Autodesk Inventor part; units mm, degrees
ref_plane "YZ Plane" through (0, 0, 0) normal (1, 0, 0) x (0, 1, 0)
ref_plane "XZ Plane" through (0, 0, 0) normal (0, 1, 0) x (-1, 0, 0)
ref_plane "XY Plane" through (0, 0, 0) normal (0, 0, 1) x (1, 0, 0)
sketch "Sketch1" plane through (0, 0, 0) normal (0, 1, 0) x (-1, 0, 0)
  line L0 (10.0011, -4.0004) -> (-4.061, -4.0004)
  line L1 (-4.061, -4.0004) -> (-4.061, -20.083)
  line L2 (-4.061, -20.083) -> (0, -13.9813)
  line L3 (0, -13.9813) -> (0, -8.1221)
  line L4 (0, -8.1221) -> (10.0011, -8.1221)
  line L5 (10.0011, -8.1221) -> (10.0011, -4.0004)
  line L6 (12.8135, 0) -> (-6.8735, 0)
  point P0 (0, 0)
revolve "Revolution1" add sketch "Sketch1" angle 360 about axis through (-10, 0, 0) along (1, 0, 0)
fillet "Fillet1" radius 2 1 edges at (4.061, 0, 20.083)
fillet "Fillet2" radius 2 2 edges at (-10.0011, 0, 8.1221) (0, 0, 8.1221)
properties part number "revolution_example"
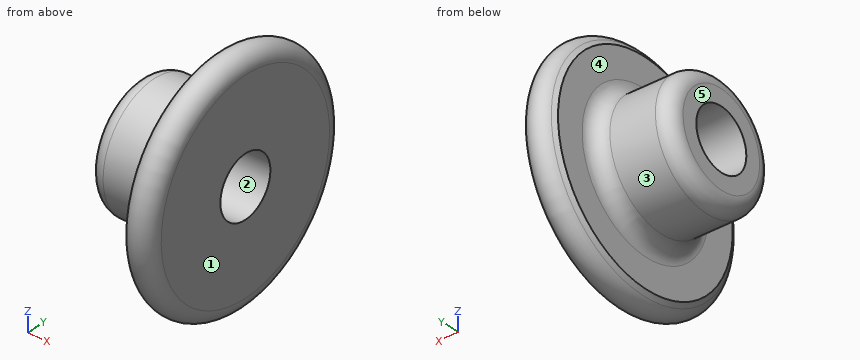
The model under review builds one solid part; all positions refer to its coordinate system, in mm. Face numbers are marked on the shaded views. A direction names the side the tool comes from. Round coordinates to 2 decimals unless told otherwise and drop trailing zeros. Write each loop counter-clockwise with the first axis right and the second up, starting at its lowest first coordinate (ties: lowest second). Pieces come first, ordered by that corner, then holes.
(1) We need section C-C on x = -3.25. Give the boundary of the cut face in (y, z), and give its area (3 significant figures).
(2) We need section D-D on x = 1. Give the boundary of the cut face in (y, z).
(3) Insertion check: pin 1 (8 mm diameter, centred on x = -8.5, y = 8, fed in from +Z); pin 2 (8 mm diameter, centred on x = -5, y = 1.5, fed in from -Z); pin 3 (4 mm diameter, centred on x = 1, y = -3, fed in from -Z). Each pin has a flat end and moves straight along its axis. Give the tip position at first contact, or say it passes through.
(4) Machinability: for the marked faces 4 and 5, which of the approach directions +Z, -Z, +X, -X, +Y, -Y give a long, thin tool a straight path to every point of the face, cutting with its end or side? Answer none if there is none.
(5) We need section A-A on y = 0. Give the boundary of the cut face in (x, z), and give its area (3 significant figures).
(6) Mouldability with a two-part tool opening along Y and no side actions: class the marked faces 1, 2 and 3 as +Y half, -Y half, draft (parallel to the pull), parting line (faces both ways), or undercut.
(7) Wall thickness on L1, parallel to Y at x = -3, z = 0; L2, parallel to X at y = -2.5, z = -11.5; L3, parallel to Y at x = -0.5, z = 0: over which ranges is each line inside the solid? List them lowest first.
Findings below:
1. outline: circle Ø16.24 at (0, 0); hole circle Ø8 at (0, 0)
1. area: 157 mm2
2. outline: circle Ø30.33 at (0, 0); hole circle Ø8 at (0, 0)
3. pin 1: stops at z = 7.05
3. pin 2: stops at z = -8.32
3. pin 3: stops at z = -15.42
4. face 4: -X
4. face 5: +Z, -Z, -X, +Y, -Y
5. outline: (-10, -6.12) arc R2 ccw to (-8, -8.12) - (-2, -8.12) arc R2 cw to (0, -10.12) - (0, -13.98) - (0.4, -14.58) arc R2 ccw to (4.06, -13.47) - (4.06, -4) - (-10, -4) - close; (-10, 4) - (4.06, 4) - (4.06, 13.47) arc R2 ccw to (0.4, 14.58) - (0, 13.98) - (0, 10.12) arc R2 cw to (-2, 8.12) - (-8, 8.12) arc R2 ccw to (-10, 6.12) - close
5. area: 172 mm2
6. face 1: draft
6. face 2: undercut
6. face 3: parting line
7. L1: y = -8.12 to -4, 4 to 8.12
7. L2: x = 0 to 4.06
7. L3: y = -8.8 to -4, 4 to 8.8
